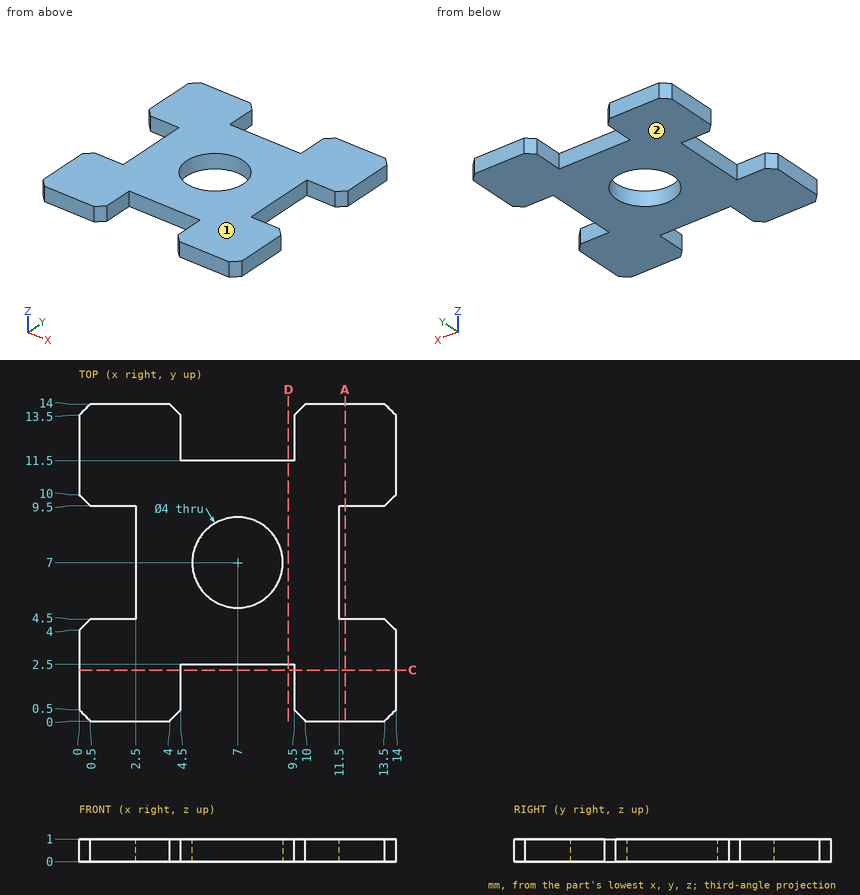
Input: dimensioned drawing with shaded views. Units: mm. Origin: part minimum x, y, z. Round coordinates to 2 decimals unless told otherwise and drop trailing zeros. Loops run counter-clockwise (first coordinate to the right, second up) from the corner with the lowest first, then second, coordinate; pieces in that order, holes last. Notation, with made-up numbers: (-24, 69) -> (34, 69) arc R34 ccw to (34, 106) -> close; hole circle Ø5 at (-7, -33). An arc over 180 degrees is marked (long way). Answer as a JSON object with one key per item and string values. Group by question number.
Q1. Mould query, pull axis Z, two halves, no side actions, for the marked faces 1 and 2. Classes: pulls with the +Z half, pulls with the -Z half, needs draft (parallel to the pull), parting line crosses it, or undercut.
Q2. Ray query, line 1 (Y direction, x = 7, z = 0.5); line 2 (X direction, y = 11.75, z = 0.4). Return the intervals inside material, ascending. Write a range as from..to.
Q3. Section query A-A (x = 11.75). Output: boundary loops of the cut face in (y, z), plus the area to 3 significant figures.
Q4. Section query D-D (x = 9.25). Output: boundary loops of the cut face in (y, z), plus the area to 3 significant figures.
Completed:
{
 "1": {"face 1": "pulls with the +Z half", "face 2": "pulls with the -Z half"},
 "2": {"line 1": "2.5..5, 9..11.5", "line 2": "0..4.5, 9.5..14"},
 "3": {"outline": "(0, 0) -> (4.5, 0) -> (4.5, 1) -> (0, 1) -> close; (9.5, 0) -> (14, 0) -> (14, 1) -> (9.5, 1) -> close", "area": "9.00 mm²"},
 "4": {"outline": "(2.5, 0) -> (11.5, 0) -> (11.5, 1) -> (2.5, 1) -> close", "area": "9.00 mm²"}
}
